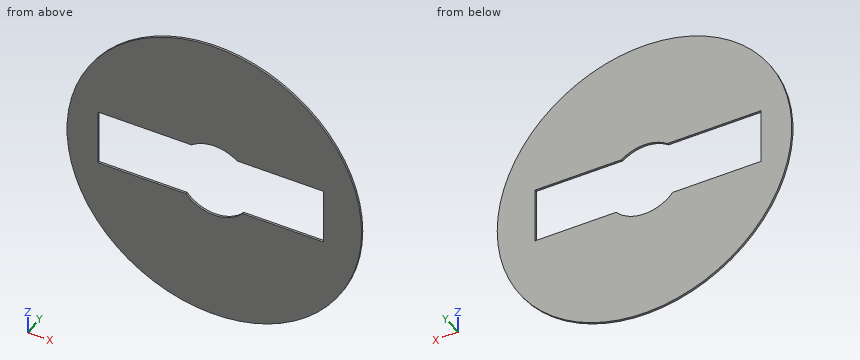
```python
from build123d import *

# Parameters (mm, degrees)
CYLINDER005_R     = 15
CYLINDER005_DEPTH = 17.84
BOX_W             = 89
BOX_H             = 17
BOX_DEPTH         = 22
CYLINDER004_R     = 58
CYLINDER004_DEPTH = 0.84


with BuildPart() as cylinder005:
    # Cylinder005 → Cylinder005 (new body)
    with BuildSketch(Plane.XZ.offset(42.6)):
        Circle(CYLINDER005_R)
    extrude(amount=CYLINDER005_DEPTH)


with BuildPart() as cube:
    # Box → Box (new body)
    with BuildSketch(Plane(origin=(-45.9, -59.6, -10), x_dir=(1, 0, 0), z_dir=(0, 0, 1))):
        with Locations((44.5, 8.5)):
            Rectangle(BOX_W, BOX_H)
    extrude(amount=BOX_DEPTH)


with BuildPart() as base:
    # Cylinder004 → Cylinder004 (new body)
    with BuildSketch(Plane.XZ.offset(49.6)):
        Circle(CYLINDER004_R)
    extrude(amount=CYLINDER004_DEPTH)

    # Cut002: cut Cube
    add(cube.part, mode=Mode.SUBTRACT)

    # Cut003: cut Cylinder005
    add(cylinder005.part, mode=Mode.SUBTRACT)


with BuildPart() as base_1:
    # Cut003 placement: moved
    add(base.part.moved(Location((0, -2, 0))))


solid = base_1.part
```
Design review of the part built by this model. Coordinates are the model's own, in mm. Give positions to 0.01 mm unless a question says otherwise; leave off trailing zeros. Write each loop counter-clockwise with the first axis right and the second up, starting at its lowest first coordinate (ties: lowest second). Pieces come first, ordered by that corner, then holes.
(1) Add section A-A (z = 0). Give the boundary of the cut face in (x, y), and give its area (3 significant figures).
Checked values:
outline: (-58, -52.44) - (-45.9, -52.44) - (-45.9, -51.6) - (-58, -51.6) - close; (43.1, -52.44) - (58, -52.44) - (58, -51.6) - (43.1, -51.6) - close
area: 22.7 mm2
(2) Add section D-D (z = 32.5). Give the boundary of the cut face in (x, y), and give its area (3 significant figures).
Checked values:
outline: (-48.04, -52.44) - (48.04, -52.44) - (48.04, -51.6) - (-48.04, -51.6) - close
area: 80.7 mm2
(3) Add section B-B (x = -42). Give the boundary of the cut face in (y, z).
Checked values:
outline: (-52.44, -40) - (-51.6, -40) - (-51.6, -10) - (-52.44, -10) - close; (-52.44, 12) - (-51.6, 12) - (-51.6, 40) - (-52.44, 40) - close
(4) Add section C-C (y = -52.2). Give the boundary of the cut face in (x, z).
Checked values:
outline: circle Ø116 at (0, 0); hole (-45.9, -10) - (-11.18, -10) arc R15 ccw to (11.18, -10) - (43.1, -10) - (43.1, 12) - (9, 12) arc R15 ccw to (-9, 12) - (-45.9, 12) - close
(5) Wall thickness on line 1 along X through (y, z) = (-51.9, -1); line 2 along Z through (x, y) = (-33.5, -52.1); line 3 along Z through (x, y) = (2, -51.9): over which ranges is each line inside the solid? List them lowest first.
Checked values:
line 1: x = -57.99 to -45.9, 43.1 to 57.99
line 2: z = -47.35 to -10, 12 to 47.35
line 3: z = -57.97 to -14.87, 14.87 to 57.97
